Read the model definition and answer for the solid it produces. Units are mm, in the model's axes. Coordinates: 2 decimals unless noted, no trailing zeros. Order: outer loops, then holes, each group sorted by start corner. A loop starts at its lowest first (then second) coordinate and runs counter-clockwise, first axis right, second up. Notation, with made-up numbers: (31, -27) -> (80, -27) arc R28 cw to (80, 9) -> close; hole circle Ø5 at (67, 14). An arc over 180 degrees is marked (long way). Use CSV: the item, a comma, the result in double quotes.
```python
from build123d import *

# Parameters (mm, degrees)
SKETCH1_R           = 1.27
BOSS_EXTRUDE1_DEPTH = 0.381
SKETCH2_W           = 2.032
SKETCH2_H           = 3.048
BOSS_EXTRUDE2_DEPTH = 0.635
CUT_EXTRUDE1_START  = -3.048
CUT_EXTRUDE1_DEPTH  = 3.048


with BuildPart() as part:
    # Sketch1 → Boss-Extrude1 (new body)
    with BuildSketch(Plane(origin=(0, 0, 0), x_dir=(1, 0, 0), z_dir=(0, 1, 0))):
        with BuildLine():
            Line((-0.695956456, 2.442794427), (-0.695956456, 2.845479033))
            Line((-0.695956456, 2.845479033), (0.695956456, 2.845479033))
            Line((0.695956456, 2.845479033), (0.695956456, 2.442794427))
            ThreePointArc((0.695956456, 2.442794427), (2.315850071, 1.043282535), (2.290753246, -1.097291924))
            Line((2.290753246, -1.097291924), (1.016, -3.758520967))
            Line((1.016, -3.758520967), (1.016, -6.806520967))
            Line((1.016, -6.806520967), (-1.016, -6.806520967))
            Line((-1.016, -6.806520967), (-1.016, -3.758520967))
            Line((-1.016, -3.758520967), (-2.290753246, -1.097291924))
            ThreePointArc((-2.290753246, -1.097291924), (-2.315850071, 1.043282535), (-0.695956456, 2.442794427))
        make_face()
        Circle(SKETCH1_R, mode=Mode.SUBTRACT)
    extrude(amount=BOSS_EXTRUDE1_DEPTH)

    # Sketch2 → Boss-Extrude2 (add)
    with BuildSketch(Plane(origin=(0, 0.381, 0), x_dir=(1, 0, 0), z_dir=(0, 1, 0))):
        with Locations((0, -5.282520967)):
            Rectangle(SKETCH2_W, SKETCH2_H)
    extrude(amount=BOSS_EXTRUDE2_DEPTH)

    # Sketch3 → Cut-Extrude1 (cut)
    with BuildSketch(Plane.XY.offset(6.806520967).offset(CUT_EXTRUDE1_START)):
        with BuildLine():
            ThreePointArc((1.016, 0.508), (0.867210245, 0.148789755), (0.508, 0))
            Line((0.508, 0), (1.016, 0))
            Line((1.016, 0), (1.016, 0.508))
        make_face()
        with BuildLine():
            ThreePointArc((-0.508, 0), (-0.867210245, 0.148789755), (-1.016, 0.508))
            Line((-1.016, 0.508), (-1.016, 0))
            Line((-1.016, 0), (-0.508, 0))
        make_face()
        with BuildLine():
            ThreePointArc((-1.016, 0.508), (-0.867210245, 0.867210245), (-0.508, 1.016))
            Line((-0.508, 1.016), (-1.016, 1.016))
            Line((-1.016, 1.016), (-1.016, 0.508))
        make_face()
        with BuildLine():
            ThreePointArc((0.105325044, 0.817704504), (0.283573941, 0.963737802), (0.508, 1.016))
            Line((0.508, 1.016), (-0.508, 1.016))
            ThreePointArc((-0.508, 1.016), (-0.283573941, 0.963737802), (-0.105325044, 0.817704504))
            Line((-0.105325044, 0.817704504), (-0.288029547, 0.635))
            ThreePointArc((-0.288029547, 0.635), (-0.727970453, 0.635), (-0.508, 0.254))
            Line((-0.508, 0.254), (0.508, 0.254))
            ThreePointArc((0.508, 0.254), (0.727970453, 0.635), (0.288029547, 0.635))
            Line((0.288029547, 0.635), (0.105325044, 0.817704504))
        make_face()
        with BuildLine():
            ThreePointArc((0.508, 1.016), (0.867210245, 0.867210245), (1.016, 0.508))
            Line((1.016, 0.508), (1.016, 1.016))
            Line((1.016, 1.016), (0.508, 1.016))
        make_face()
    extrude(amount=CUT_EXTRUDE1_DEPTH, mode=Mode.SUBTRACT)


solid = part.part
```
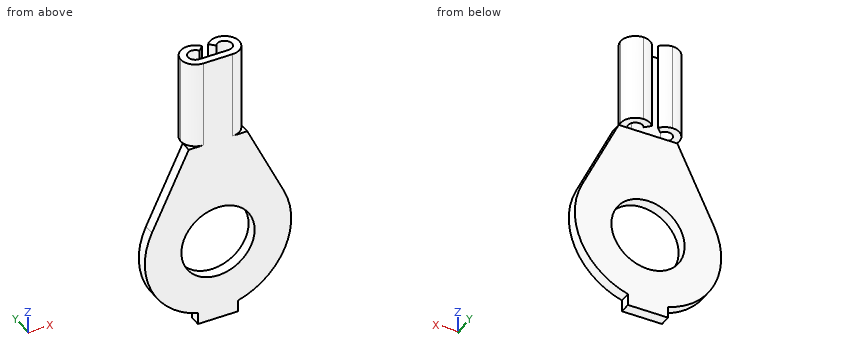
Item 1: Straight lines are drawn through the part: line 1 along X through (y, z) = (0.2, 0); line 2 along Y through (x, z) = (0.5, 6.5); line 3 along Y through (x, z) = (-0.9, 2.25). For each, find the intervals that lie inside material, in ascending order.
Return value:
line 1,"x = -2.54 to -1.27, 1.27 to 2.54"
line 2,"y = 0 to 0.25, 0.76 to 1.02"
line 3,"y = 0 to 0.38"
Item 2: Find section A-A, the plane x = 0. Give the vertices of the cut face in (y, z).
Return value:
outline,"(0, -2.85) -> (0.38, -2.85) -> (0.38, -1.27) -> (0, -1.27) -> close; (0, 1.27) -> (0.38, 1.27) -> (0.38, 3.76) -> (0.25, 3.76) -> (0.25, 6.81) -> (0, 6.81) -> close"
Item 3: Each of these flat-tipped pins is pushed along its axis until it touches: P1, Ø0.8, axis at x = 0, z = 5, coming from the +Y side; P2, Ø1.5, axis at x = 2, z = 1.5, coming from the +Y side. Where does it stop, or does it pass through?
Return value:
P1,"stops at y = 1"
P2,"stops at y = 0.38"
Item 4: Find section B-B, the plane z = 0. Give the vertices of the cut face in (x, y), then the cut area to 3 significant figures.
Return value:
outline,"(-2.54, 0) -> (-1.27, 0) -> (-1.27, 0.38) -> (-2.54, 0.38) -> close; (1.27, 0) -> (2.54, 0) -> (2.54, 0.38) -> (1.27, 0.38) -> close"
area,"0.968 mm^2"
Item 5: Find section C-C, the plane z = 5. Give the vertices of the cut face in (x, y) (3 decimals).
Return value:
outline,"(-0.508, 0) -> (0.508, 0) arc R0.508 ccw (long way) to (0.105, 0.818) -> (0.288, 0.635) arc R0.254 cw (long way) to (0.508, 0.254) -> (-0.508, 0.254) arc R0.254 cw (long way) to (-0.288, 0.635) -> (-0.105, 0.818) arc R0.508 ccw (long way) to start"
Item 6: Find section D-D, the plane y = 0.15. Give the vertices of the cut face in (x, z).
Return value:
outline,"(-2.29, 1.1) arc R2.54 ccw to (-0.7, -2.44) -> (-0.7, -2.85) -> (0.7, -2.85) -> (0.7, -2.44) arc R2.54 ccw to (2.29, 1.1) -> (1.02, 3.76) -> (0.87, 3.76) -> (0.87, 6.81) -> (-0.87, 6.81) -> (-0.87, 3.76) -> (-1.02, 3.76) -> close; hole circle Ø2.54 at (0, 0)"
